Model file for the job. Use its own axes, mm. Face numbers are marked on the shaded views. A direction names the side the tool comes from. Round coordinates to 2 decimals unless told otherwise and drop trailing zeros. Order: outer loops, then holes, each group sorted by start corner. A loop starts at its lowest first (then second) coordinate and runs counter-clockwise, first axis right, second up. Notation, with made-up numbers: (44, 76) - (89, 76) arc R7 cw to (89, 82) - close; hole circle Ø5 at (89.5, 59.25). An arc over 180 degrees is marked (long way). Write item = value, one per line. Start each with the question number.
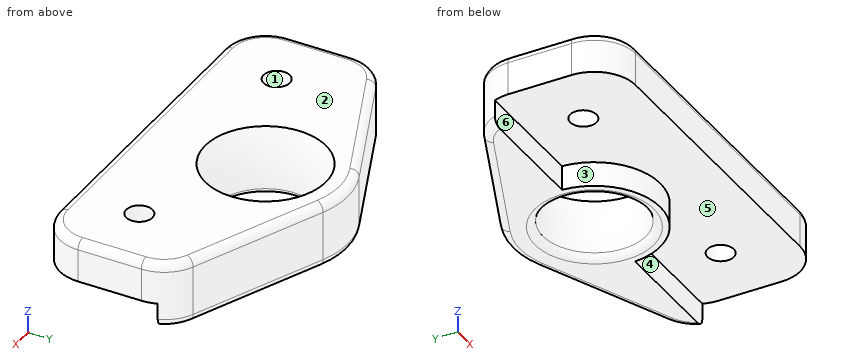
from build123d import *

# Parameters (mm, degrees)
ESQUISSE1_R             = 1.6
BOSS_EXTRU_1_DEPTH      = 8
ESQUISSE2_W             = 3
ESQUISSE2_H             = 14.5
ENL_V_MAT_EXTRU_1_DEPTH = 50.040799341
ESQUISSE5_R             = 8
BOSS_EXTRU_2_DEPTH      = 3
CONG_1_R                = 5
CONG_2_R                = 1


with BuildPart() as part:
    # Esquisse1 → Boss.-Extru.1 (new body)
    with BuildSketch(Plane.XY):
        with BuildLine():
            Line((-23, 1), (-3.948369031, 9.187512285))
            ThreePointArc((-3.948369031, 9.187512285), (0, 10), (3.948369031, 9.187512285))
            Line((3.948369031, 9.187512285), (23, 1))
            Line((23, 1), (23, -15))
            Line((23, -15), (-23, -15))
            Line((-23, -15), (-23, 1))
        make_face()
        with Locations((-15, -7)):
            Circle(ESQUISSE1_R, mode=Mode.SUBTRACT)
        with Locations(Location((15, -7, 0), (0, 0, 180))):
            Circle(ESQUISSE1_R, mode=Mode.SUBTRACT)
    extrude(amount=BOSS_EXTRU_1_DEPTH)

    # Esquisse2 → Enlèv. mat.-Extru.1 (cut, through all)
    with BuildSketch(Plane(origin=(23, 0, 0), x_dir=(0, 0, -1), z_dir=(1, 0, 0))):
        with Locations((-1.5, -7.75)):
            Rectangle(ESQUISSE2_W, ESQUISSE2_H)
    extrude(amount=-ENL_V_MAT_EXTRU_1_DEPTH, mode=Mode.SUBTRACT)

    # Esquisse5 → Boss.-Extru.2 (add)
    with BuildSketch(Plane(origin=(0, 0, 0), x_dir=(-1, 0, 0), z_dir=(0, 0, -1))):
        Circle(ESQUISSE5_R)
    extrude(amount=-BOSS_EXTRU_2_DEPTH)

    # Esquisse4 → Enlèvement de matière-Révolution1 (revolve, cut)
    with BuildSketch(Plane(origin=(0, 0, 0), x_dir=(0, 0, -1), z_dir=(1, 0, 0)), mode=Mode.PRIVATE) as enl_vement_de_mati_re_r_volution1_sk:
        with BuildLine():
            Line((-8, 0), (0, 0))
            Line((0, 0), (0, 6.460607986))
            ThreePointArc((0, 6.460607986), (-4.092346509, 6.059840087), (-8, 7.339745962))
            Line((-8, 7.339745962), (-8, 0))
        make_face()
    revolve(enl_vement_de_mati_re_r_volution1_sk.sketch.rotate(Axis((0, 0, 8), (0, 0, -1)), 90), axis=Axis((0, 0, 8), (0, 0, -1)), mode=Mode.SUBTRACT)

    # Congé1
    cong_1_edges = [part.edges().sort_by_distance(p)[0] for p in [
        (-23, -15, 5.5),
        (-23, 1, 4),
        (23, -15, 5.5),
        (23, 1, 4),
    ]]
    fillet(cong_1_edges, radius=CONG_1_R)

    # Congé2
    cong_2_edges = [part.edges().sort_by_distance(p)[0] for p in [
        (0, 10, 8),
        (-11.961276773, 5.743934112, 8),
        (-6.460607986, 0, 0),
        (-11.961276773, 5.743934112, 0),
        (0, -15, 8),
        (0, 10, 0),
        (-23, -6.146700103, 8),
        (23, -6.146700103, 8),
        (11.961276773, 5.743934112, 8),
        (22.175579156, 0.456970445, 8),
        (21.535533906, -13.535533906, 8),
        (-22.175579156, 0.456970445, 8),
        (-21.535533906, -13.535533906, 8),
        (11.961276773, 5.743934112, 0),
        (21.60386416, 1.17245656, 0),
        (-21.60386416, 1.17245656, 0),
    ]]
    fillet(cong_2_edges, radius=CONG_2_R)


solid = part.part
Item 1: Mould opens along X. For the marked faces 1, 2 and 3 say: +X half, -X half, draft (parallel to the pull), parting line (faces both ways), or undercut.
Item 2: Saw through at C-C, the plane z = 6. Give the cut face in (x, y), then the cut area to 3 significant figures.
Item 3: Which spindle directions (+Z, -Z, +X, -X, +Y, -Y) get a long thin tool onto all of the face, cutting with end or side? Do the marked faces 4, 5 and 6. Say none if no direction does.
Item 4: Drop flat-ended pins along their axis: pin 1 (1.5 mm diameter, centred on y = -0.5, z = 4.5, fed in from -X); pin 2 (3.5 mm diameter, centred on x = -14.5, z = 1, fed in from -Y); pin 3 (3 mm diameter, centred on x = 15, y = -7, fed in from -Z); pin 4 (5 mm diameter, centred on x = -15, y = -7, fed in from -Z). Give the stop position or say it passes through.
Item 5: Probe L1, parallel to X at y = -7, z = 6.2; L2, parallel to X at y = -7.75, z = 6; L3, parallel to Z at x = 7, y = -11.5. List the from-to ranges inside material, lowest first.
Item 6: Saw through at B-B, the plane z = 1.75. Give the cut face in (x, y).
Item 7: Saw through at A-A, the plane z = 3.75. Give the cut face in (x, y).
Check sheet entries:
q1.face_1 = undercut
q1.face_2 = draft
q1.face_3 = parting line
q2.outline = (-23, -10) arc R5 ccw to (-18, -15) - (18, -15) arc R5 ccw to (23, -10) - (23, -2.29) arc R5 ccw to (19.97, 2.3) - (3.95, 9.19) arc R10 ccw to (-3.95, 9.19) - (-19.97, 2.3) arc R5 ccw to (-23, -2.29) - close; hole circle Ø3.2 at (-15, -7); hole circle Ø12.92 at (0, 0); hole circle Ø3.2 at (15, -7)
q2.area = 799 mm2
q3.face_4 = -Z, +X, -Y
q3.face_5 = -Z, -Y
q3.face_6 = -Z, -X, -Y
q4.pin_1 = -22.89
q4.pin_2 = -0.5
q4.pin_3 = through
q4.pin_4 = 3
q5.L1 = -23 to -16.6, -13.4 to 13.4, 16.6 to 23
q5.L2 = -23 to -16.41, -13.59 to 13.59, 16.41 to 23
q5.L3 = 3 to 8
q6.outline = (-22.67, -0.5) - (-7.98, -0.5) arc R8 ccw to (7.98, -0.5) - (22.67, -0.5) arc R5 ccw to (19.97, 2.3) - (3.95, 9.19) arc R10 ccw to (-3.95, 9.19) - (-19.97, 2.3) arc R5 ccw to start; hole circle Ø12.16 at (0, 0)
q7.outline = (-23, -10) arc R5 ccw to (-18, -15) - (18, -15) arc R5 ccw to (23, -10) - (23, -2.29) arc R5 ccw to (19.97, 2.3) - (3.95, 9.19) arc R10 ccw to (-3.95, 9.19) - (-19.97, 2.3) arc R5 ccw to (-23, -2.29) - close; hole circle Ø3.2 at (-15, -7); hole circle Ø12.06 at (0, 0); hole circle Ø3.2 at (15, -7)
